Could you check a few things on this model? Use its own coordinates, in mm. Face numbers are marked on the shaded views. Coordinates: 2 decimals unless noted, no trailing zeros. One line per item, written item: value. Start each with the question number.
(1) I'm going to push flat-ended pins straight in: P1, Ø1, axis at y = -4, z = 3, coming from the +X side; P2, Ø1, axis at x = 10.45, y = 0, coming from the -Z side; P3, Ø3, axis at y = -21, z = 2, coming from the -X side; P4, Ø1, axis at x = 23.5, z = 4.5, coming from the -Y side. Where does each tip first touch, or does it pass through?
(2) If we mould it in two halves opening along X, with no side actions, what happens to the marked faces 1, 2 and 3? For each: pulls with the +X half, pulls with the -X half, needs draft (parallel to the pull), parting line crosses it, or undercut.
(3) If I drill on line 1 along Y through (x, z) = (0, 4.9); line 2 along X through (y, z) = (-13.5, 0.5); line 3 along Y through (x, z) = (16, 4.75), over which ranges is the centre line in solid material (lowest first)? Write a range as from..to.
(4) If we section it at A-A on z = 4: Count the separate pieces of the cut face and the enclosed holes in it, then the cut area to 3 significant figures.
```python
from build123d import *

# Parameters (mm, degrees)
ESQUISSE2_R             = 30
ESQUISSE2_R_2           = 0.6
ESQUISSE2_R_3           = 2.4
ESQUISSE2_R_4           = 7.692251906
BOSS_EXTRU_1_DEPTH      = 6
ENL_V_MAT_EXTRU_1_DEPTH = 2


with BuildPart() as part:
    # Esquisse2 → Boss.-Extru.1 (new body)
    with BuildSketch(Plane.XY):
        Circle(ESQUISSE2_R)
        with Locations((0, 10.45)):
            Circle(ESQUISSE2_R_2, mode=Mode.SUBTRACT)
        with Locations((0, 6.45)):
            Circle(ESQUISSE2_R_2, mode=Mode.SUBTRACT)
        Circle(ESQUISSE2_R_3, mode=Mode.SUBTRACT)
        with Locations((10.45, 0)):
            Circle(ESQUISSE2_R_2, mode=Mode.SUBTRACT)
        with Locations((6.45, 0)):
            Circle(ESQUISSE2_R_2, mode=Mode.SUBTRACT)
        with Locations((0, -10.45)):
            Circle(ESQUISSE2_R_2, mode=Mode.SUBTRACT)
        with Locations((0, -6.45)):
            Circle(ESQUISSE2_R_2, mode=Mode.SUBTRACT)
        with Locations((-10.45, 0)):
            Circle(ESQUISSE2_R_2, mode=Mode.SUBTRACT)
        with Locations((-6.45, 0)):
            Circle(ESQUISSE2_R_2, mode=Mode.SUBTRACT)
        with Locations((-12.727922061, 12.727922061)):
            Circle(ESQUISSE2_R_4, mode=Mode.SUBTRACT)
        with Locations((12.727922061, 12.727922061)):
            Circle(ESQUISSE2_R_4, mode=Mode.SUBTRACT)
        with Locations((12.727922061, -12.727922061)):
            Circle(ESQUISSE2_R_4, mode=Mode.SUBTRACT)
        with Locations((-12.727922061, -12.727922061)):
            Circle(ESQUISSE2_R_4, mode=Mode.SUBTRACT)
    extrude(amount=BOSS_EXTRU_1_DEPTH)

    # Esquisse3 → Enlèv. mat.-Extru.1 (cut)
    with BuildSketch(Plane(origin=(0, 0, 0), x_dir=(-1, 0, 0), z_dir=(0, 0, -1))):
        with BuildLine():
            Line((-2.530820261, -4.390158503), (-1.99702088, -14.159121967))
            ThreePointArc((-1.99702088, -14.159121967), (0, -16.05), (1.99702088, -14.159121967))
            Line((1.99702088, -14.159121967), (2.530820261, -4.390158503))
            ThreePointArc((2.530820261, -4.390158503), (3.583192911, -3.583192911), (4.390158503, -2.530820261))
            Line((4.390158503, -2.530820261), (14.159121967, -1.99702088))
            ThreePointArc((14.159121967, -1.99702088), (16.05, 0), (14.159121967, 1.99702088))
            Line((14.159121967, 1.99702088), (4.390158503, 2.530820261))
            ThreePointArc((4.390158503, 2.530820261), (3.583192911, 3.583192911), (2.530820261, 4.390158503))
            Line((2.530820261, 4.390158503), (1.99702088, 14.159121967))
            ThreePointArc((1.99702088, 14.159121967), (0, 16.05), (-1.99702088, 14.159121967))
            Line((-1.99702088, 14.159121967), (-2.530820261, 4.390158503))
            ThreePointArc((-2.530820261, 4.390158503), (-3.583192911, 3.583192911), (-4.390158503, 2.530820261))
            Line((-4.390158503, 2.530820261), (-14.159121967, 1.99702088))
            ThreePointArc((-14.159121967, 1.99702088), (-16.05, 0), (-14.159121967, -1.99702088))
            Line((-14.159121967, -1.99702088), (-4.390158503, -2.530820261))
            ThreePointArc((-4.390158503, -2.530820261), (-3.583192911, -3.583192911), (-2.530820261, -4.390158503))
        make_face()
    extrude(amount=-ENL_V_MAT_EXTRU_1_DEPTH, mode=Mode.SUBTRACT)

    # Enlèvement de matière-Balayage1: sweep along a curve in space
    with BuildLine() as enl_vement_de_mati_re_balayage1_path:
        ThreePointArc((30, 0, 0), (21.213203436, 21.213203436, 0), (0, 30, 0))
        ThreePointArc((0, 30, 0), (-21.213203436, 21.213203436, 0), (-30, 0, 0))
        ThreePointArc((-30, 0, 0), (-21.213203436, -21.213203436, 0), (0, -30, 0))
        ThreePointArc((0, -30, 0), (21.213203436, -21.213203436, 0), (30, 0, 0))
    # Esquisse4 → Enlèvement de matière-Balayage1 (sweep, cut)
    with BuildSketch(Plane(origin=(0, 0, 0), x_dir=(1, 0, 0), z_dir=(0, 1, 0))):
        Polygon((-31.389656083, -5.473341376), (-27.521569936, -3.290275959), (-31.389656083, -0.638208742), align=None)
    sweep(path=enl_vement_de_mati_re_balayage1_path.line, mode=Mode.SUBTRACT)


solid = part.part
```
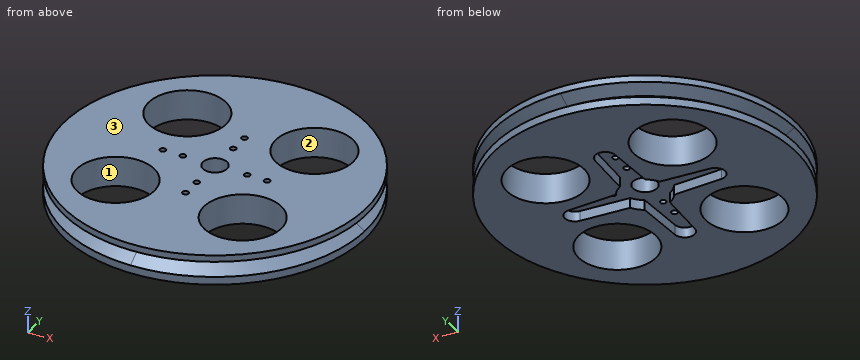
Values:
1. P1: stops at x = 28.4
1. P2: passes through
1. P3: stops at x = -22.75
1. P4: stops at y = -19.22
2. face 1: undercut
2. face 2: undercut
2. face 3: needs draft
3. line 1: y = -30..-11.05, -9.85..-7.05, -5.85..-2.4, 2.4..5.85, 7.05..9.85, 11.05..30
3. line 2: x = -26.79..-20.38, -5.07..-2.03, 2.03..5.07, 20.38..26.79
3. line 3: y = -25.38..-19.69, -5.77..5.77, 19.69..25.38
4. separate pieces: 1
4. enclosed holes: 13
4. area: 1,830 mm2
